Check sheet for the drawn part. Datum: minimum x, y, z corner. Units: mm. A direction names the side the tool comes from. Coordinates: 2 decimals unless noted, no trailing zeros. Write each loop counter-clockwise with the first axis right and the second up, starting at its lowest first coordinate (ties: lowest second). Pieces come first, ordered by that corner, then holes. Notation, with made-up numbers: (-29.75, -24.75) - (0.25, -24.75) arc R16 ccw to (0.25, -7.75) - close; hole circle Ø2 at (13, -9). An arc over 180 degrees is marked (long way). Use one line per item in the form item = value. Start each with the question number.
1. Cross-section at C-C on x = 7.25. Record the boundary of the cut face in (y, z) (1 decimal), then the cut area to 3 significant figures.
2. Go/stop test with flat-tipped pins: pin 1 Ø1 at (x, y) = (11, 8) entering from +Z (1 decimal); pin 2 Ø4 at (x, y) = (11, 4.5) entering from -Z; pin 3 Ø2 at (y, z) = (17, 8) entering from -X (1 decimal); pin 4 Ø2 at (x, y) = (1.5, 2) entering from +Z. Record where each tip stops, or that it passes through.
3. Tool access check on the marked faces 1, 2, 3 and 4. Record the directions out of +Z, -Z, +X, -X, +Y, -Y that give a thin tool (end or side, any length) a straight path to the whole face; none if there is none.
4. Draft check along Z on the marked faces 5, 6 and 7. Enter one of: +Z half, -Z half, draft (parallel to the pull), parting line (faces both ways), or undercut.
5. Cross-section at B-B on z = 6.5. Record the boundary of the cut face in (x, y), then the cut area to 3 significant figures.
6. Scan lines: line 1 along Y through (x, z) = (3.5, 13.75); line 2 along X through (y, z) = (4.75, 7.5); line 3 along Z through (x, y) = (6.75, 5). Record each from-to range of solid material in increasing order.
7. Cross-section at D-D on x = 1.5. Record the boundary of the cut face in (y, z).
8. Cross-section at A-A on y = 17.75. Record the boundary of the cut face in (x, z) (1 decimal), then the cut area to 3 significant figures.
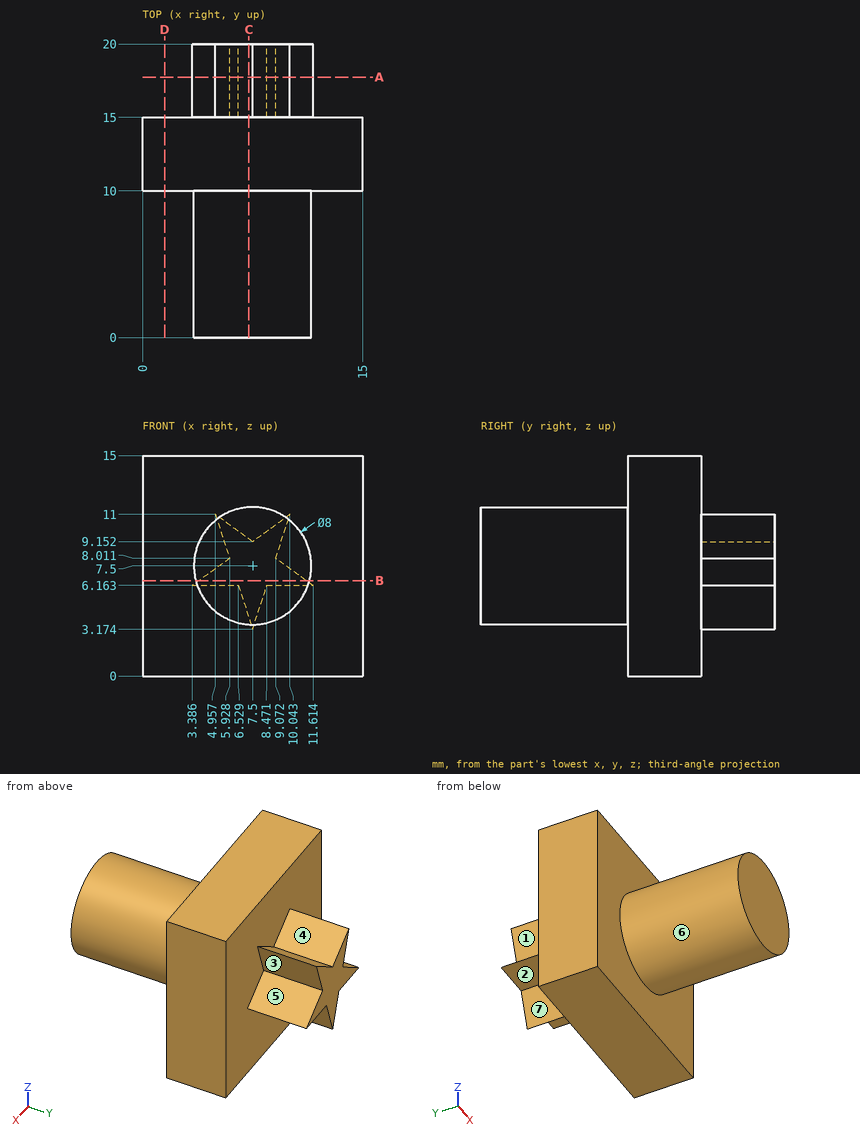
Final values:
q1.outline = (0, 3.5) - (10, 3.5) - (10, 0) - (15, 0) - (15, 3.9) - (20, 3.9) - (20, 9.3) - (15, 9.3) - (15, 15) - (10, 15) - (10, 11.5) - (0, 11.5) - close
q1.area = 182 mm²
q2.pin_1 = 10.1
q2.pin_2 = 3.79
q2.pin_3 = 4.5
q2.pin_4 = through
q3.face_1 = -X, +Y
q3.face_2 = -Z, -X, +Y
q3.face_3 = +X, +Y
q3.face_4 = +Z, +Y
q4.face_5 = undercut
q4.face_6 = parting line
q4.face_7 = -Z half
q5.outline = (0, 10) - (3.63, 10) - (3.63, 0) - (11.37, 0) - (11.37, 10) - (15, 10) - (15, 15) - (11.15, 15) - (11.15, 20) - (3.85, 20) - (3.85, 15) - (0, 15) - close
q5.area = 189 mm²
q6.line_1 = 10 to 15
q6.line_2 = 3.5 to 11.5
q6.line_3 = 3.57 to 11.43
q7.outline = (10, 0) - (15, 0) - (15, 15) - (10, 15) - close
q8.outline = (3.4, 6.2) - (6.5, 6.2) - (7.5, 3.2) - (8.5, 6.2) - (11.6, 6.2) - (9.1, 8) - (10, 11) - (7.5, 9.2) - (5, 11) - (5.9, 8) - close
q8.area = 21.0 mm²
